Source: three-view drawing plus pictorial views. Frame: mm from the lowest corner of the part. Give positions to 0.01 mm unless a question says otherwise; leave off trailing zeros. Write each loop counter-clockwise with the first axis right and the second up, starting at its lowest first coordinate (ties: lowest second). Pieces come first, ordered by that corner, then holes.
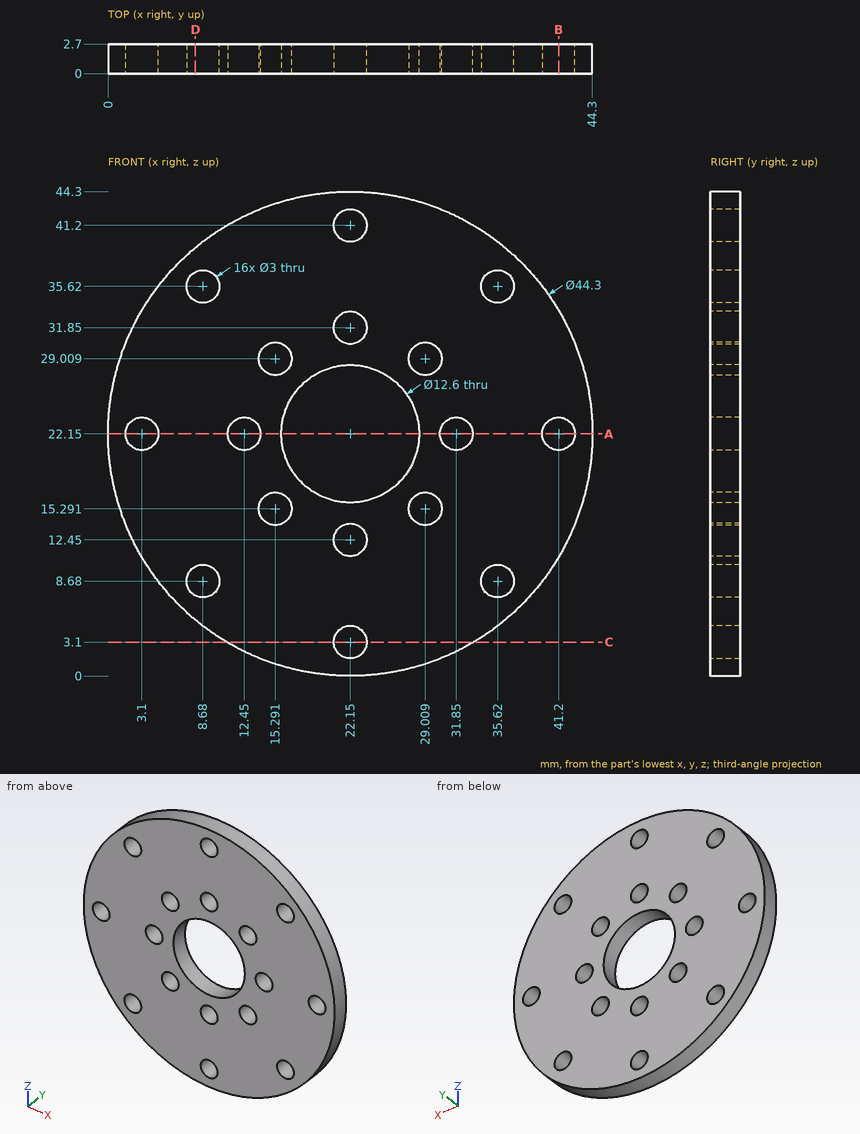
Q1. Section A-A on z = 22.15. Output: boundary loops of the cut face in (x, y).
Filled sheet:
outline: (0, 0) - (1.6, 0) - (1.6, 2.7) - (0, 2.7) - close; (4.6, 0) - (10.95, 0) - (10.95, 2.7) - (4.6, 2.7) - close; (13.95, 0) - (15.85, 0) - (15.85, 2.7) - (13.95, 2.7) - close; (28.45, 0) - (30.35, 0) - (30.35, 2.7) - (28.45, 2.7) - close; (33.35, 0) - (39.7, 0) - (39.7, 2.7) - (33.35, 2.7) - close; (42.7, 0) - (44.3, 0) - (44.3, 2.7) - (42.7, 2.7) - close
Q2. Section B-B on x = 41.2. Output: boundary loops of the cut face in (y, z).
Filled sheet:
outline: (0, 10.85) - (2.7, 10.85) - (2.7, 20.65) - (0, 20.65) - close; (0, 23.65) - (2.7, 23.65) - (2.7, 33.45) - (0, 33.45) - close
Q3. Section C-C on z = 3.1. Output: boundary loops of the cut face in (x, y).
Filled sheet:
outline: (10.85, 0) - (20.65, 0) - (20.65, 2.7) - (10.85, 2.7) - close; (23.65, 0) - (33.45, 0) - (33.45, 2.7) - (23.65, 2.7) - close
Q4. Ray query, line 1 along Z through (x, y) = (22, 1.5); line 2 along X through (y, z) = (1.65, 22.15); line 3 along Z through (x, y) = (9.5, 0.6) (1 decimal). Return the intervals inside material, ascending.
Filled sheet:
line 1: z = 0 to 1.61, 4.59 to 10.96, 13.94 to 15.85, 28.45 to 30.36, 33.34 to 39.71, 42.69 to 44.3
line 2: x = 0 to 1.6, 4.6 to 10.95, 13.95 to 15.85, 28.45 to 30.35, 33.35 to 39.7, 42.7 to 44.3
line 3: z = 4 to 7.4, 9.9 to 34.4, 36.9 to 40.3
Q5. Section D-D on x = 8. Output: boundary loops of the cut face in (y, z).
Filled sheet:
outline: (0, 5.11) - (2.7, 5.11) - (2.7, 7.34) - (0, 7.34) - close; (0, 10.02) - (2.7, 10.02) - (2.7, 34.28) - (0, 34.28) - close; (0, 36.96) - (2.7, 36.96) - (2.7, 39.19) - (0, 39.19) - close
Q6. Pin query (flat end, axial travel): P1, Ø2.5, axis at x = 35.62, z = 8.68, coming from the +Y side; P2, Ø1.5, axis at y = 1, z = 26, coming from the +X side; P3, Ø1.5, axis at x = 26.5, y = 1, coming from the -Z side (1 decimal). Return the tip coordinate at first contact, or that it passes through.
Filled sheet:
P1: passes through
P2: stops at x = 44.08
P3: stops at z = 0.3
